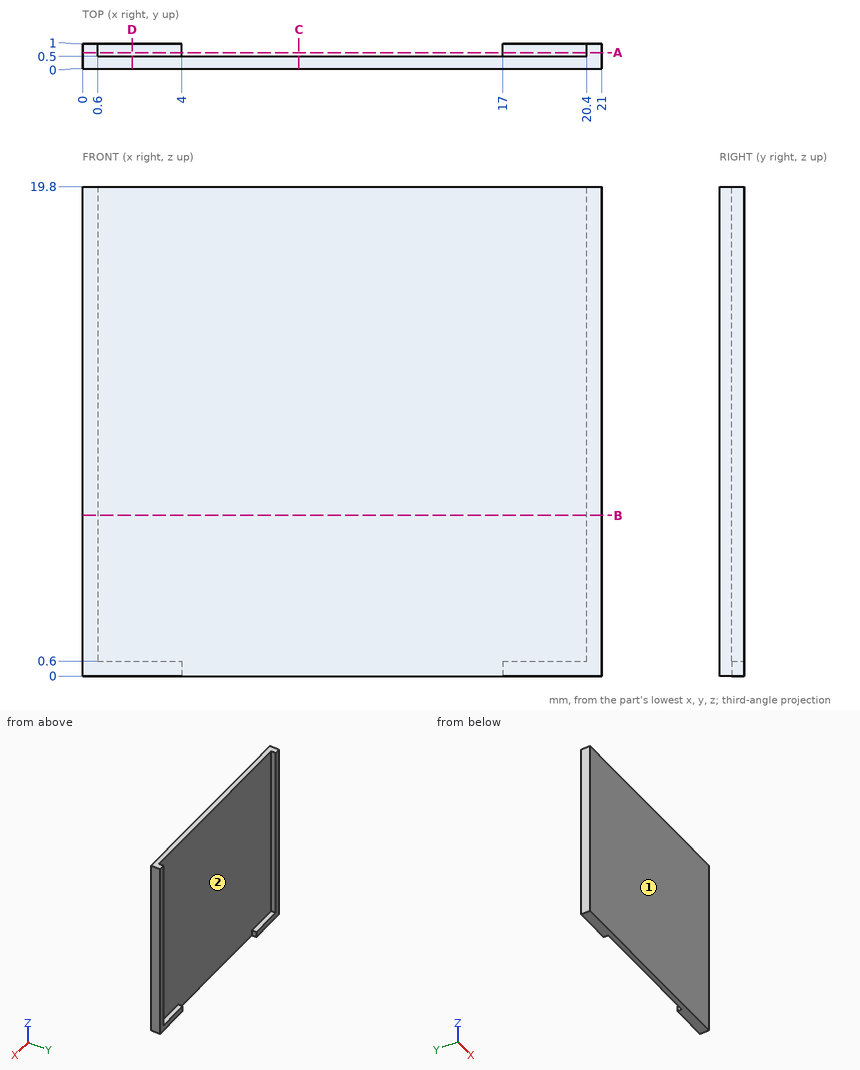
Can you work these out from the drawing? Everything is in mm from the part's minimum corner. Coordinates: 2 decimals unless noted, no trailing zeros. Order: outer loops, then holes, each group sorted by start corner. A loop starts at its lowest first (then second) coordinate and runs counter-clockwise, first axis right, second up. Notation, with made-up numbers: (52.25, 36) -> (70.25, 36) arc R14 ccw to (70.25, 57) -> close; hole circle Ø7 at (55.5, -19.75). An arc over 180 degrees is marked (long way). Return JSON: item names as keys, results as strings.
1) If we section it at D-D on x = 2: List the corners of the cut face in (y, z) for me, plus the area to 3 significant figures.
Conclusion:
{"outline": "(0, 0) -> (1, 0) -> (1, 0.6) -> (0.5, 0.6) -> (0.5, 19.8) -> (0, 19.8) -> close", "area": "10.2 mm²"}
2) I'm going to push a flat-ended pin straight in: P1, Ø10, axis at x = 13, z = 10, coming from the +Y side. Where does the tip first touch, or does it pass through?
Conclusion:
{"P1": "stops at y = 0.5"}
3) If we section it at B-B on z = 6.5: List the corners of the cut face in (x, y) for me, plus the area to 3 significant figures.
Conclusion:
{"outline": "(0, 0) -> (21, 0) -> (21, 1) -> (20.4, 1) -> (20.4, 0.5) -> (0.6, 0.5) -> (0.6, 1) -> (0, 1) -> close", "area": "11.1 mm²"}
4) If I drill on probe 1 along X at (y, z) = (0.55, 10.25); probe 2 along Y at (x, z) = (18, 18); probe 3 along Z at (x, y) = (17.75, 0.95), over which ranges is the centre line in solid material (lowest first)?
Conclusion:
{"probe 1": "x = 0 to 0.6, 20.4 to 21", "probe 2": "y = 0 to 0.5", "probe 3": "z = 0 to 0.6"}
5) If we section it at A-A on y = 0.65: List the corners of the cut face in (x, z) for me.
Conclusion:
{"outline": "(0, 0) -> (4, 0) -> (4, 0.6) -> (0.6, 0.6) -> (0.6, 19.8) -> (0, 19.8) -> close; (17, 0) -> (21, 0) -> (21, 19.8) -> (20.4, 19.8) -> (20.4, 0.6) -> (17, 0.6) -> close"}
6) If we section it at C-C on x = 8.75: List the corners of the cut face in (y, z) for me.
Conclusion:
{"outline": "(0, 0) -> (0.5, 0) -> (0.5, 19.8) -> (0, 19.8) -> close"}
7) Thinking about a two-plate mould opening in X: for the marked faces 1 and 2, which applies, +X half, -X half, draft (parallel to the pull), parting line (faces both ways), or undercut?
Conclusion:
{"face 1": "draft", "face 2": "undercut"}
